Geometry check sheet. Reference: the model listing, model coordinates, mm. Face numbers are marked on the shaded views. A direction names the side the tool comes from. Give positions to 0.01 mm unless a question says otherwise; leave off trailing zeros. Order: outer loops, then holes, each group sorted by start corner. A loop starts at its lowest first (then second) coordinate and runs counter-clockwise, first axis right, second up. Notation, with made-up numbers: M 81.5,2 L 85.5,2 A32 cw 85.5,35 Z; hole C -9.5,-2 d7. An arc over 180 degrees is marked long. Answer as a JSON object with one key per item and string values. Group by question number.
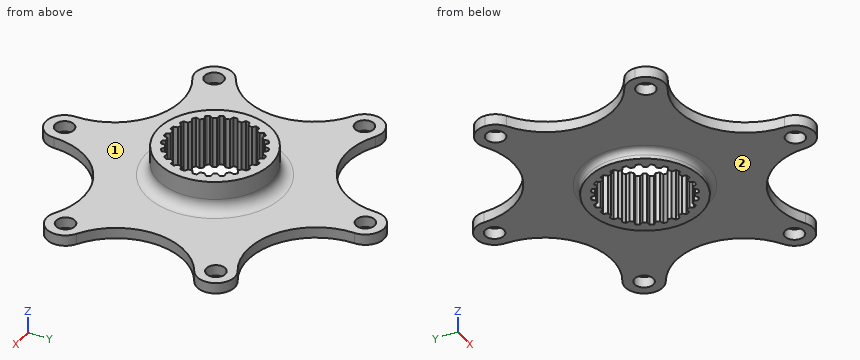
from build123d import *

# Parameters (mm, degrees)
SKETCH1_R           = 115
BOSS_EXTRUDE1_DEPTH = 13.55
CUT_EXTRUDE1_DEPTH  = 165.87695412
SKETCH3_R           = 95
SKETCH3_R_2         = 30
CUT_EXTRUDE13_DEPTH = 16.06
FILLET1_R           = 6.35
CUT_EXTRUDE14_START = -5.27
SKETCH7_R           = 95
SKETCH7_R_2         = 30
CUT_EXTRUDE14_DEPTH = 5.27
FILLET2_R           = 3.175
SKETCH8_R           = 115
SKETCH8_R_2         = 95
CUT_EXTRUDE17_DEPTH = 165.87695412
SKETCH9_R           = 5
CUT_EXTRUDE20_DEPTH = 10
SKETCH10_R          = 95
CUT_EXTRUDE21_DEPTH = 10


with BuildPart() as part:
    # Sketch1 → Boss-Extrude1 (new, symmetric)
    with BuildSketch(Plane.XY):
        with Locations(Location((0, 0, 0), (0, 0, 180))):
            Circle(SKETCH1_R)
    extrude(amount=BOSS_EXTRUDE1_DEPTH, both=True)

    # Sketch2 → Cut-Extrude1 (cut, through all)
    with BuildSketch(Plane.XY.offset(13.55)):
        Polygon((1.065531645, 23.075412075), (-1.065531645, 23.075412075), (-2.179683155, 25.005179098), (-3.276207429, 24.885266027), (-4.366404331, 24.717291793), (-4.943131584, 22.564916358), (-7.001580653, 22.013356593), (-8.577228822, 23.589004771), (-9.605354152, 23.189376274), (-10.614928564, 22.744961902), (-10.614928564, 20.516658882), (-12.460483511, 19.451127237), (-14.390250527, 20.565278751), (-15.27991187, 19.913168849), (-16.140062965, 19.222600444), (-15.563335705, 17.070225009), (-17.070225009, 15.563335705), (-19.22260044, 16.140062971), (-19.913168845, 15.279911875), (-20.565278747, 14.390250533), (-19.451127237, 12.460483511), (-20.516658882, 10.614928564), (-22.744961899, 10.614928571), (-23.189376271, 9.605354159), (-23.589004769, 8.577228829), (-22.013356593, 7.001580653), (-22.564916358, 4.943131584), (-24.717291793, 4.366404331), (-24.885266027, 3.276207429), (-25.005179098, 2.179683155), (-23.075412075, 1.065531645), (-23.075412075, -1.065531645), (-25.005179098, -2.179683148), (-24.885266028, -3.276207422), (-24.717291794, -4.366404324), (-22.564916358, -4.943131584), (-22.013356593, -7.001580653), (-23.589004771, -8.577228822), (-23.189376274, -9.605354152), (-22.744961902, -10.614928564), (-20.516658882, -10.614928564), (-19.451127237, -12.460483511), (-20.565278751, -14.390250527), (-19.913168849, -15.27991187), (-19.222600444, -16.140062965), (-17.070225009, -15.563335705), (-15.563335705, -17.070225009), (-16.140062971, -19.22260044), (-15.279911875, -19.913168845), (-14.390250533, -20.565278747), (-12.460483511, -19.451127237), (-10.614928564, -20.516658882), (-10.614928571, -22.744961899), (-9.605354159, -23.189376271), (-8.577228829, -23.589004769), (-7.001580653, -22.013356593), (-4.943131584, -22.564916358), (-4.366404331, -24.717291793), (-3.276207429, -24.885266027), (-2.179683155, -25.005179098), (-1.065531645, -23.075412075), (1.065531645, -23.075412075), (2.179683148, -25.005179098), (3.276207422, -24.885266028), (4.366404324, -24.717291794), (4.943131584, -22.564916358), (7.001580653, -22.013356593), (8.577228822, -23.589004771), (9.605354152, -23.189376274), (10.614928564, -22.744961902), (10.614928564, -20.516658882), (12.460483511, -19.451127237), (14.390250527, -20.565278751), (15.27991187, -19.913168849), (16.140062965, -19.222600444), (15.563335705, -17.070225009), (17.070225009, -15.563335705), (19.22260044, -16.140062971), (19.913168845, -15.279911875), (20.565278747, -14.390250533), (19.451127237, -12.460483511), (20.516658882, -10.614928564), (22.744961899, -10.614928571), (23.189376271, -9.605354159), (23.589004769, -8.577228829), (22.013356593, -7.001580653), (22.564916358, -4.943131584), (24.717291793, -4.366404331), (24.885266027, -3.276207429), (25.005179098, -2.179683155), (23.075412075, -1.065531645), (23.075412075, 1.065531645), (25.005179098, 2.179683148), (24.885266028, 3.276207422), (24.717291794, 4.366404324), (22.564916358, 4.943131584), (22.013356593, 7.001580653), (23.589004771, 8.577228822), (23.189376274, 9.605354152), (22.744961902, 10.614928564), (20.516658882, 10.614928564), (19.451127237, 12.460483511), (20.565278751, 14.390250527), (19.913168849, 15.27991187), (19.222600444, 16.140062965), (17.070225009, 15.563335705), (15.563335705, 17.070225009), (16.140062971, 19.22260044), (15.279911876, 19.913168845), (14.390250533, 20.565278747), (12.460483511, 19.451127237), (10.614928564, 20.516658882), (10.614928571, 22.744961899), (9.605354159, 23.189376271), (8.577228829, 23.589004769), (7.001580653, 22.013356593), (4.943131584, 22.564916358), (4.366404331, 24.717291793), (3.276207429, 24.885266027), (2.179683155, 25.005179098), align=None)
    extrude(amount=-CUT_EXTRUDE1_DEPTH, mode=Mode.SUBTRACT)

    # Sketch3 → Cut-Extrude13 (cut)
    with BuildSketch(Plane.XY.offset(13.55)):
        Circle(SKETCH3_R)
        Circle(SKETCH3_R_2, mode=Mode.SUBTRACT)
    extrude(amount=-CUT_EXTRUDE13_DEPTH, mode=Mode.SUBTRACT)

    # Fillet1
    fillet1_edges = [part.edges().sort_by_distance(p)[0] for p in [
        (-30, 0, -2.51),
    ]]
    fillet(fillet1_edges, radius=FILLET1_R)

    # Sketch7 → Cut-Extrude14 (cut)
    with BuildSketch(Plane(origin=(0, 0, -13.55), x_dir=(-1, 0, 0), z_dir=(0, 0, -1)).offset(CUT_EXTRUDE14_START)):
        with Locations(Location((0, 0, 0), (0, 0, 180))):
            Circle(SKETCH7_R)
        with Locations(Location((0, 0, 0), (0, 0, 180))):
            Circle(SKETCH7_R_2, mode=Mode.SUBTRACT)
    extrude(amount=CUT_EXTRUDE14_DEPTH, mode=Mode.SUBTRACT)

    # Fillet2
    fillet2_edges = [part.edges().sort_by_distance(p)[0] for p in [
        (-30, 0, -8.28),
    ]]
    fillet(fillet2_edges, radius=FILLET2_R)

    # Sketch8 → Cut-Extrude17 (cut, through all)
    with BuildSketch(Plane(origin=(0, 0, -13.55), x_dir=(-1, 0, 0), z_dir=(0, 0, -1))):
        Circle(SKETCH8_R)
        Circle(SKETCH8_R_2, mode=Mode.SUBTRACT)
    extrude(amount=-CUT_EXTRUDE17_DEPTH, mode=Mode.SUBTRACT)

    # Sketch9 → Cut-Extrude20 (cut)
    with BuildSketch(Plane(origin=(0, 0, -8.28), x_dir=(-1, 0, 0), z_dir=(0, 0, -1))):
        with Locations((0, 80)):
            Circle(SKETCH9_R)
        with Locations((69.282032303, 40)):
            Circle(SKETCH9_R)
        with Locations((69.282032303, -40)):
            Circle(SKETCH9_R)
        with Locations((0, -80)):
            Circle(SKETCH9_R)
        with Locations((-69.282032303, -40)):
            Circle(SKETCH9_R)
        with Locations((-69.282032303, 40)):
            Circle(SKETCH9_R)
    extrude(amount=-CUT_EXTRUDE20_DEPTH, mode=Mode.SUBTRACT)

    # Sketch10 → Cut-Extrude21 (cut)
    with BuildSketch(Plane(origin=(0, 0, -8.28), x_dir=(-1, 0, 0), z_dir=(0, 0, -1))):
        Circle(SKETCH10_R)
        with BuildLine():
            ThreePointArc((-74.282032303, 31.339745962), (-77.942286341, 45), (-64.282032303, 48.660254038))
            ThreePointArc((-64.282032303, 48.660254038), (-28.094011813, 48.660255848), (-10, 80))
            ThreePointArc((-10, 80), (0, 90), (10, 80))
            ThreePointArc((10, 80), (28.094011813, 48.660255848), (64.282032303, 48.660254038))
            ThreePointArc((64.282032303, 48.660254038), (74.282032303, 48.660254038), (79.282032303, 40))
            ThreePointArc((79.282032303, 40), (77.942286341, 35), (74.282032303, 31.339745962))
            ThreePointArc((74.282032303, 31.339745962), (56.188023625, 0), (74.282032303, -31.339745962))
            ThreePointArc((74.282032303, -31.339745962), (77.942286341, -35), (79.282032303, -40))
            ThreePointArc((79.282032303, -40), (74.282032303, -48.660254038), (64.282032303, -48.660254038))
            ThreePointArc((64.282032303, -48.660254038), (28.094011813, -48.660255848), (10, -80))
            ThreePointArc((10, -80), (0, -90), (-10, -80))
            ThreePointArc((-10, -80), (-28.094011813, -48.660255848), (-64.282032303, -48.660254038))
            ThreePointArc((-64.282032303, -48.660254038), (-77.942286341, -45), (-74.282032303, -31.339745962))
            ThreePointArc((-74.282032303, -31.339745962), (-56.188023625, 0), (-74.282032303, 31.339745962))
        make_face(mode=Mode.SUBTRACT)
    extrude(amount=-CUT_EXTRUDE21_DEPTH, mode=Mode.SUBTRACT)


solid = part.part
1. Depth check by flat-ended pin: pin 1 (1 mm diameter, centred on x = 17.5, z = -7, fed in from +Y); pin 2 (6 mm diameter, centred on y = -5, z = 10.5, fed in from -X); pin 3 (1.8 mm diameter, centred on x = 21.5, z = 0.5, fed in from -Y). Enter the tip coordinate at first touch or a pass-through.
2. Thickness scan on line 1 along Y through (x, z) = (-0.5, 11); line 2 along X through (y, z) = (19.5, -8.25); line 3 along Y through (x, z) = (-2, -7.5). Record the ranges inside material, lowest first. Write a range as [from, to].
3. Cross-section at A-A (x = 67.5). Record the cut outline in (y, z).
4. Access from +Z, -Z, +X, -X, +Y, -Y to the whole of each face (thin tool, end or side, straight path). Record for the marked faces 1 and 2.
5. Cross-section at B-B (x = 46). Record the cut outline in (y, z).
Report:
{
 "1": {"pin 1": "stops at y = 58.61", "pin 2": "stops at x = -29.93", "pin 3": "stops at y = -23.47"},
 "2": {"line 1": "y = [-30, -23.08], [23.08, 30]", "line 2": "x = [-61.89, -15.79], [-12.55, -12.38], [12.38, 12.55], [15.79, 61.89]", "line 3": "y = [-89.8, -84.58], [-75.42, -24.69], [24.69, 75.42], [84.58, 89.8]"},
 "3": {"outline": "M -49.84,-8.28 L -44.67,-8.28 L -44.67,-2.51 L -49.84,-2.51 Z; M -35.33,-8.28 L -26.28,-8.28 L -26.28,-2.51 L -35.33,-2.51 Z; M 26.28,-8.28 L 35.33,-8.28 L 35.33,-2.51 L 26.28,-2.51 Z; M 44.67,-8.28 L 49.84,-8.28 L 49.84,-2.51 L 44.67,-2.51 Z"},
 "4": {"face 1": "+Z", "face 2": "-Z"},
 "5": {"outline": "M -43.81,-8.28 L 43.81,-8.28 L 43.81,-2.51 L -43.81,-2.51 Z"}
}
